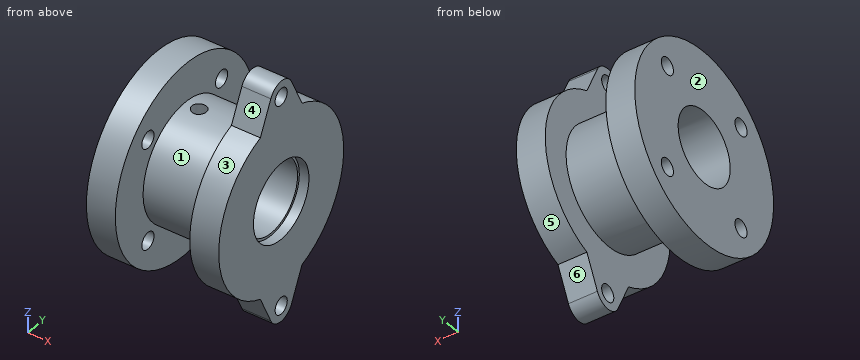
```python
from build123d import *

# Parameters (mm, degrees)
SKETCH1_R               = 20
SKETCH1_R_2             = 7.5
BOSS_EXTRUDE1_DEPTH     = 6
SKETCH3_R               = 12
SKETCH3_R_2             = 7.5
BOSS_EXTRUDE2_DEPTH     = 14
CUT_EXTRUDE2_DEPTH      = 35.641016151
CUT_EXTRUDE2_DEPTH_BACK = 35.641016151
SKETCH4_R               = 1.5
SKETCH5_R               = 18
SKETCH5_R_2             = 7.5
BOSS_EXTRUDE3_DEPTH     = 6
BOSS_EXTRUDE4_START     = -6
SKETCH6_R               = 1.75
BOSS_EXTRUDE4_DEPTH     = 6
SKETCH2_R               = 1.75
CUT_EXTRUDE1_DEPTH      = 6
SKETCH7_R               = 8
CUT_EXTRUDE3_DEPTH      = 2


with BuildPart() as part:
    # Sketch1 → Boss-Extrude1 (new body)
    with BuildSketch(Plane(origin=(0, 0, 0), x_dir=(0, 0, -1), z_dir=(1, 0, 0))):
        Circle(SKETCH1_R)
        Circle(SKETCH1_R_2, mode=Mode.SUBTRACT)
    extrude(amount=BOSS_EXTRUDE1_DEPTH)

    # Sketch3 → Boss-Extrude2 (add)
    with BuildSketch(Plane(origin=(6, 0, 0), x_dir=(0, 0, -1), z_dir=(1, 0, 0))):
        Circle(SKETCH3_R)
        Circle(SKETCH3_R_2, mode=Mode.SUBTRACT)
    extrude(amount=BOSS_EXTRUDE2_DEPTH)

    # Sketch4 → Cut-Extrude2 (cut, two sides: drawn at the far end of the back side and taken through both)
    with BuildSketch(Plane.XY.offset(-CUT_EXTRUDE2_DEPTH_BACK)):
        with Locations((9, 0)):
            Circle(SKETCH4_R)
    extrude(amount=CUT_EXTRUDE2_DEPTH + CUT_EXTRUDE2_DEPTH_BACK, mode=Mode.SUBTRACT)

    # Sketch5 → Boss-Extrude3 (add)
    with BuildSketch(Plane(origin=(20, 0, 0), x_dir=(0, 0, -1), z_dir=(1, 0, 0))):
        Circle(SKETCH5_R)
        Circle(SKETCH5_R_2, mode=Mode.SUBTRACT)
    extrude(amount=BOSS_EXTRUDE3_DEPTH)

    # Sketch6 → Boss-Extrude4 (add)
    # profile 1 of 2: a face of its own
    with BuildSketch(Plane(origin=(26, 0, 0), x_dir=(0, 0, -1), z_dir=(1, 0, 0)).offset(BOSS_EXTRUDE4_START)):
        with BuildLine():
            Line((-23.358800107, 2.984171955), (-16.970562748, 6))
            ThreePointArc((-16.970562748, 6), (-18, 0), (-16.970562748, -6))
            Line((-16.970562748, -6), (-23.358800107, -2.984171955))
            ThreePointArc((-23.358800107, -2.984171955), (-25.25, 0), (-23.358800107, 2.984171955))
        make_face()
        with Locations((-21.95, 0)):
            Circle(SKETCH6_R, mode=Mode.SUBTRACT)
    # profile 2 of 2: a face of its own
    with BuildSketch(Plane(origin=(26, 0, 0), x_dir=(0, 0, -1), z_dir=(1, 0, 0)).offset(BOSS_EXTRUDE4_START)):
        with BuildLine():
            Line((23.358800107, 2.984171955), (16.970562748, 6))
            ThreePointArc((16.970562748, 6), (18, 0), (16.970562748, -6))
            Line((16.970562748, -6), (23.358800107, -2.984171955))
            ThreePointArc((23.358800107, -2.984171955), (25.25, 0), (23.358800107, 2.984171955))
        make_face()
        with Locations((21.95, 0)):
            Circle(SKETCH6_R, mode=Mode.SUBTRACT)
    extrude(amount=BOSS_EXTRUDE4_DEPTH)

    # Sketch2 → Cut-Extrude1 (cut)
    with BuildSketch(Plane.ZY):
        with Locations((-10.606601718, 10.606601718)):
            Circle(SKETCH2_R)
        with Locations((10.606601718, 10.606601718)):
            Circle(SKETCH2_R)
        with Locations((10.606601718, -10.606601718)):
            Circle(SKETCH2_R)
        with Locations((-10.606601718, -10.606601718)):
            Circle(SKETCH2_R)
    extrude(amount=-CUT_EXTRUDE1_DEPTH, mode=Mode.SUBTRACT)

    # Sketch7 → Cut-Extrude3 (cut)
    with BuildSketch(Plane(origin=(26, 0, 0), x_dir=(0, 0, -1), z_dir=(1, 0, 0))):
        Circle(SKETCH7_R)
    extrude(amount=-CUT_EXTRUDE3_DEPTH, mode=Mode.SUBTRACT)


solid = part.part
```
Work out the finished part from the listing and answer in its coordinate system (mm). Face numbers are marked on the shaded views. A direction names the side the tool comes from. Coordinates: 2 decimals unless noted, no trailing zeros. Loops run counter-clockwise (first coordinate to the right, second up) from the corner with the lowest first, then second, coordinate; pieces in that order, holes last. Notation, with made-up numbers: M 43.5,70 L 77.5,70 A14 cw 77.5,74 Z; hole C -32,-16.75 d10. An arc over 180 degrees is marked long. Use CSV: the item, a comma, the result in double quotes. Start each with the question number.
(1) Find section A-A, the plane z = 0. Give the vertices of the cut face in (x, y).
(2) For the marked faces 4, 5 and 6, determine the directions among +Z, -Z, +X, -X, +Y, -Y from which every point of the face is accessible in a straight line to the end or side of a thin tool.
(3) Find section D-D, the plane x = 9.75. Give the vertices of the cut face in (y, z), then the cut area to 3 significant figures.
(4) Given pin 1 Ø3.5 at (x, y) = (9, 0) entering from +Z; pin 2 Ø6 at (x, y) = (5, 7.5) entering from +Z; pin 3 Ø2 at (y, z) = (10.61, -10.61) entering from -X, each flat-ended and moving along its own axis, determine where each tip first touches the part or whether it passes through.
(5) Find section B-B, the plane x = 23. Give the vertices of the cut face in (y, z).
(6) Find section C-C, the plane z = -10. Give the vertices of the cut face in (x, y).
(7) For a pull along X with two mould halves and no side action, classify the marked faces 1, 2 and 3 as +X half, -X half, draft (parallel to the pull), parting line (faces both ways), or undercut.
(8) Consider line 1 (X direction, y = 7.5, z = -10); line 2 (Z direction, x = 6.25, y = 0); line 3 (X direction, y = -2.5, z = 22.5). Determine where each line is inside the solid, lowest interval first.
Recorded:
1,outline,"M 0,-20 L 6,-20 L 6,-12 L 20,-12 L 20,-18 L 26,-18 L 26,-8 L 24,-8 L 24,-7.5 L 0,-7.5 Z; M 0,7.5 L 24,7.5 L 24,8 L 26,8 L 26,18 L 20,18 L 20,12 L 6,12 L 6,20 L 0,20 Z"
2,face 4,"+Z, +X, -Y"
2,face 5,"+X, +Y"
2,face 6,"-Z, +X, +Y"
3,outline,"M -1.3,-11.93 L -1.3,-7.39 A7.5 cw -1.3,7.39 L -1.3,11.93 A12 ccw Z; M 1.3,-11.93 A12 ccw 1.3,11.93 L 1.3,7.39 A7.5 cw 1.3,-7.39 Z"
3,area,"252 mm^2"
4,pin 1,"stops at z = 12"
4,pin 2,"stops at z = 19.49"
4,pin 3,"stops at x = 20"
5,outline,"M -6,-16.97 L -2.98,-23.36 A3.3 ccw 2.98,-23.36 L 6,-16.97 A18 ccw 6,16.97 L 2.98,23.36 A3.3 ccw -2.98,23.36 L -6,16.97 A18 ccw Z; hole C 0,0 d15; hole C 0,-21.95 d3.5; hole C 0,21.95 d3.5"
6,outline,"M 0,-17.32 L 6,-17.32 L 6,-12.25 L 0,-12.25 Z; M 0,-8.97 L 6,-8.97 L 6,-6.63 L 20,-6.63 L 20,-14.97 L 26,-14.97 L 26,14.97 L 20,14.97 L 20,6.63 L 6,6.63 L 6,8.97 L 0,8.97 Z; M 0,12.25 L 6,12.25 L 6,17.32 L 0,17.32 Z; hole C 9,0 d3"
7,face 1,"undercut"
7,face 2,"-X half"
7,face 3,"draft"
8,line 1,"x = 0 to 6, 20 to 26"
8,line 2,"z = -12 to -7.5, 7.5 to 12"
8,line 3,"x = 20 to 26"
